The listing builds one solid part. Answer for the finished solid, in the listing's coordinates (mm). Face numbers are marked on the shaded views. A direction names the side the tool comes from. Round coordinates to 2 decimals unless told otherwise and drop trailing zeros. Loops run counter-clockwise (first coordinate to the right, second up) from the corner with the lowest first, then second, coordinate; pieces in that order, holes last. Notation, with made-up numbers: (77.5, -16.5) -> (115.5, -16.5) arc R32 ccw to (115.5, 13.5) -> close; hole circle Ø4 at (5, 1). An arc over 180 degrees is marked (long way). Use a Markdown table: item, result. Add a question column.
Q1. Consider line 1 (X direction, y = 10, z = 0); line 2 (X direction, y = 45, z = 0); line 3 (Z direction, x = 0, y = 16). Determine where each line is inside the solid, lowest interval first.
Q2. Given pin 1 Ø8 at (x, y) = (4, 30) entering from +Z; pin 2 Ø0.8 at (x, y) = (22, 44) entering from -Z; pin 3 Ø0.8 at (x, z) = (22, -6.5) entering from -Y; pin 4 Ø0.5 at (x, y) = (-22, 42.5) entering from +Z, each flat-ended and moving along its own axis, determine where each tip first touches the part or whether it passes through.
Q3. Which of the six approach directions +Z, -Z, +X, -X, +Y, -Y give full straight-line access (tool end or side, diameter ignored) to the marked faces 4, 5 and 6?
Q4. Section A-A on z = 0 is taken. Give the vertices of the cut face in (x, y).
Q5. For a pull along Y with two mould halves and no side action, classify the marked faces 1, 2 and 3 as released by +Y, released by -Y, zero draft, split by the parting line, or undercut.
Q6. Section D-D on z = -10 is taken. Give the vertices of the cut face in (x, y).
Q7. Section B-B on x = 0 is taken. Give the vertices of the cut face in (y, z).
Q8. Section C-C on y = 7.5 is taken. Give the vertices of the cut face in (x, z).
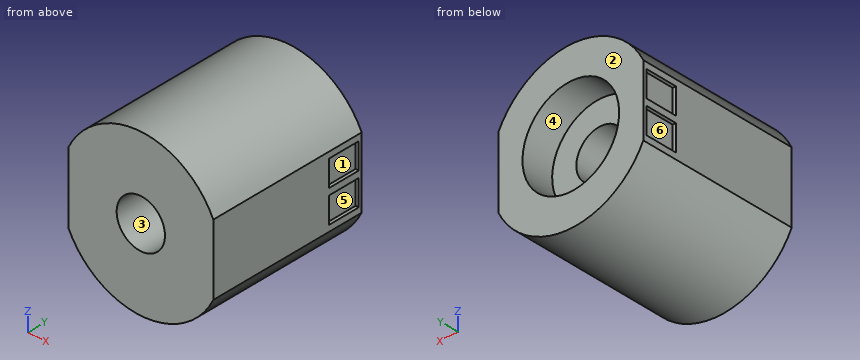
from build123d import *

# Parameters (mm, degrees)
SKETCH_1_R          = 25
SKETCH_1_R_2        = 7.5
EXTRUDE_1_DEPTH     = 50
SKETCH_2_R          = 15
CUT_EXTRUDE_1_DEPTH = 10
SKETCH_3_OUTSIDE_W  = 69.32
SKETCH_3_OUTSIDE_H  = 69.32
CUT_EXTRUDE_2_DEPTH = 62.23724357
SKETCH_4_W          = 8
SKETCH_4_H          = 10
CUT_EXTRUDE_3_DEPTH = 1


with BuildPart() as part:
    # ｽｹｯﾁ1 → ﾎﾞｽ - 押し出し1 (new body)
    with BuildSketch(Plane(origin=(0, 0, 0), x_dir=(1, 0, 0), z_dir=(0, 1, 0))):
        with Locations(Location((0, 0, 0), (0, 0, 270))):
            Circle(SKETCH_1_R)
        with Locations(Location((0, 0, 0), (0, 0, 270))):
            Circle(SKETCH_1_R_2, mode=Mode.SUBTRACT)
    extrude(amount=EXTRUDE_1_DEPTH)

    # ｽｹｯﾁ2 → ｶｯﾄ - 押し出し1 (cut)
    with BuildSketch(Plane(origin=(0, 50, 0), x_dir=(1, 0, 0), z_dir=(0, 1, 0))):
        with Locations(Location((0, 0, 0), (0, 0, 270))):
            Circle(SKETCH_2_R)
    extrude(amount=-CUT_EXTRUDE_1_DEPTH, mode=Mode.SUBTRACT)

    # ｽｹｯﾁ3 outside → ｶｯﾄ - 押し出し2 (cut, through all)
    with BuildSketch(Plane(origin=(0, 50, 0), x_dir=(1, 0, 0), z_dir=(0, 1, 0))):
        Rectangle(SKETCH_3_OUTSIDE_W, SKETCH_3_OUTSIDE_H)
        with BuildLine():
            Line((-22.5, 10.897247359), (-22.5, -10.897247359))
            ThreePointArc((-22.5, -10.897247359), (0, -25), (22.5, -10.897247359))
            Line((22.5, -10.897247359), (22.5, 10.897247359))
            ThreePointArc((22.5, 10.897247359), (0, 25), (-22.5, 10.897247359))
        make_face(mode=Mode.SUBTRACT)
    extrude(amount=-CUT_EXTRUDE_2_DEPTH, mode=Mode.SUBTRACT)

    # ｽｹｯﾁ4 → ｶｯﾄ - 押し出し3 (cut)
    with BuildSketch(Plane.ZY.offset(22.5)):
        with Locations((-5, 44)):
            Rectangle(SKETCH_4_W, SKETCH_4_H)
        with Locations((5, 44)):
            Rectangle(SKETCH_4_W, SKETCH_4_H)
    cut_extrude_3 = extrude(amount=-CUT_EXTRUDE_3_DEPTH, mode=Mode.SUBTRACT)

    # ﾐﾗｰ1: ｶｯﾄ - 押し出し3 across plane
    add(cut_extrude_3.mirror(Plane(origin=(0, 0, 0), x_dir=(0, 0, 1), z_dir=(1, 0, 0))), mode=Mode.SUBTRACT)


solid = part.part
Checked values:
| question | item | result |
|---|---|---|
| 1 | line 1 | x = -22.5 to -7.5, 7.5 to 22.5 |
| 1 | line 2 | x = -22.5 to -15, 15 to 22.5 |
| 1 | line 3 | z = -25 to -7.5, 7.5 to 25 |
| 2 | pin 1 | stops at z = 25 |
| 2 | pin 2 | stops at z = -12.59 |
| 2 | pin 3 | stops at y = 0 |
| 2 | pin 4 | stops at z = 12.33 |
| 3 | face 4 | +Y |
| 3 | face 5 | +X |
| 3 | face 6 | -X |
| 4 | outline | (-22.5, 0) -> (-7.5, 0) -> (-7.5, 40) -> (-15, 40) -> (-15, 50) -> (-22.5, 50) -> close; (7.5, 0) -> (22.5, 0) -> (22.5, 50) -> (15, 50) -> (15, 40) -> (7.5, 40) -> close |
| 5 | face 1 | undercut |
| 5 | face 2 | released by +Y |
| 5 | face 3 | zero draft |
| 6 | outline | (-22.5, 0) -> (22.5, 0) -> (22.5, 50) -> (11.18, 50) -> (11.18, 40) -> (-11.18, 40) -> (-11.18, 50) -> (-22.5, 50) -> close |
| 7 | outline | (0, -25) -> (50, -25) -> (50, -15) -> (40, -15) -> (40, -7.5) -> (0, -7.5) -> close; (0, 7.5) -> (40, 7.5) -> (40, 15) -> (50, 15) -> (50, 25) -> (0, 25) -> close |
| 8 | outline | (-22.5, -10.9) arc R25 ccw to (22.5, -10.9) -> (22.5, 10.9) arc R25 ccw to (-22.5, 10.9) -> close; hole circle Ø15 at (0, 0) |
